The model under review builds one solid part; all positions refer to its coordinate system, in mm. A direction names the side the tool comes from. Give positions to 0.01 mm unless a question says otherwise; leave off trailing zeros. Order: outer loops, then holes, each group sorted by start corner. A loop starts at its lowest first (then second) coordinate and runs counter-clockwise, first axis right, second up.
```python
from build123d import *

# Parameters (mm, degrees)
ESQUISSE1_W                     = 10.5
ESQUISSE1_H                     = 1.75
ESQUISSE2_R                     = 4.45
BOSS_EXTRU_1_DEPTH              = 2.5
ESQUISSE3_R                     = 3.75
BOSS_EXTRU_2_DEPTH              = 0.5
DIAM_TRE_DU_PER_AGE_1_5_1_5_1_D = 1.5


with BuildPart() as part:
    # Esquisse1 → Révolution1 (revolve)
    with BuildSketch(Plane(origin=(0, 0, 0), x_dir=(-1, 0, 0), z_dir=(0, 0, -1)), mode=Mode.PRIVATE) as r_volution1_sk:
        with Locations((-5.25, -0.875)):
            Rectangle(ESQUISSE1_W, ESQUISSE1_H)
    revolve(r_volution1_sk.sketch.rotate(Axis((0, -1.75, 0), (0, 1, 0)), 270), axis=Axis((0, -1.75, 0), (0, 1, 0)))

    # Esquisse2 → Boss.-Extru.1 (add)
    with BuildSketch(Plane.XZ.offset(1.75)):
        with Locations(Location((0, 0, 0), (0, 0, 270))):
            Circle(ESQUISSE2_R)
    extrude(amount=BOSS_EXTRU_1_DEPTH)

    # Esquisse3 → Boss.-Extru.2 (add)
    with BuildSketch(Plane(origin=(0, 0, 0), x_dir=(-1, 0, 0), z_dir=(0, 1, 0))):
        with Locations(Location((0, 0, 0), (0, 0, 90))):
            Circle(ESQUISSE3_R)
    extrude(amount=BOSS_EXTRU_2_DEPTH)

    # Esquisse4 → Enlèvement de matière-Révolution1 (revolve, cut)
    with BuildSketch(Plane(origin=(0, 0, 0), x_dir=(-1, 0, 0), z_dir=(0, 0, -1)), mode=Mode.PRIVATE) as enl_vement_de_mati_re_r_volution1_sk:
        Polygon((-3, -4.5), (0, -4.5), (0, 0.5), (-3, 0.5), (-3, -0.5), (-1.500593113, -0.5), (-1.500593113, -1.5), (-3, -1.5), align=None)
    revolve(enl_vement_de_mati_re_r_volution1_sk.sketch.rotate(Axis((0, -4.5, 0), (0, 1, 0)), 270), axis=Axis((0, -4.5, 0), (0, 1, 0)), mode=Mode.SUBTRACT)

    # Diamètre du perçage Ø1.5 (1.5)1 (through all)
    with Locations(Plane(origin=(0, -1.75, 0), x_dir=(-1, 0, 0), z_dir=(0, -1, 0))):
        with Locations((-7, 0), (0, 7), (7, 0), (0, -7)):
            Hole(DIAM_TRE_DU_PER_AGE_1_5_1_5_1_D / 2)


solid = part.part
```
Item 1: Draft analysis for pull direction Z (two halves, no side actions). For faces 1 (the cylindrical face through (0.9, -0.01, 2.86)), 2 (the flat face through (3, 0.5, 1)), 3 (the cylindrical face through (3.01, -2.98, 3.28)), 4 (the flat face through (-1.3, -1.5, -1.3)), state which applies: released by +Z, released by -Z, zero draft, split by the parting line, or undercut.
Values found:
face 1: undercut
face 2: zero draft
face 3: split by the parting line
face 4: undercut
Item 2: Take a section at A-A (z = 0). Give the number of separate pieces and of enclosed holes in the cut face, and give its area (3 significant figures).
Values found:
separate pieces: 4
enclosed holes: 0
area: 32.0 mm2
Item 3: For line 1 (Z direction, x = 0.5, y = -1.4); line 2 (Y direction, x = 2.5, z = 8.5); line 3 (X direction, y = -2, z = 0), list the stretches that pass through material, from the lowest coordinate up.
Values found:
line 1: z = -10.49 to -7.56, -6.44 to -1.41, 1.41 to 6.44, 7.56 to 10.49
line 2: y = -1.75 to 0
line 3: x = -4.45 to -3, 3 to 4.45
Item 4: Clearance check with flat-ended pins moving along their axes: pin 1 Ø1.5 at (x, y) = (3.5, -1.5) entering from +Z; pin 2 Ø6 at (x, z) = (-7.5, 2.5) entering from -Y; pin 3 Ø5 at (x, z) = (0, 0) entering from +Y. State where each tip first meets the part, or that it passes through.
Values found:
pin 1: stops at z = 10.13
pin 2: stops at y = -1.75
pin 3: stops at y = -0.5
Item 5: Take a section at B-B (x = 6.5). Give the boundary of the cut face in (y, z), and give its area (3 significant figures).
Values found:
outline: (-1.75, -8.25) - (0, -8.25) - (0, -0.56) - (-1.75, -0.56) - close; (-1.75, 0.56) - (0, 0.56) - (0, 8.25) - (-1.75, 8.25) - close
area: 26.9 mm2
Item 6: Take a section at C-C (y = -1.1). Give the boundary of the cut face in (x, z), and give its area (3 significant figures).
Values found:
outline: circle Ø21 at (0, 0); hole circle Ø1.5 at (-7, 0); hole circle Ø3 at (0, 0); hole circle Ø1.5 at (0, -7); hole circle Ø1.5 at (0, 7); hole circle Ø1.5 at (7, 0)
area: 332 mm2
Item 7: For faces 5 (the flat face through (0, 0, 5)), 6 (the flat face through (0, -1.75, 5)), 7 (the cylindrical face through (3.2, -0.9, 10)), list the 3-axis set-ups (+Z, -Z, +X, -X, +Y, -Y) from which the entire face can be reached by the end or side of a thin tool; tool diameter is ignored.
Values found:
face 5: +Y
face 6: -Y
face 7: +Y, -Y
Item 8: Take a section at D-D (y = -3.55). Give the boundary of the cut face in (x, z), and give its area (3 significant figures).
Values found:
outline: circle Ø8.9 at (0, 0); hole circle Ø6 at (0, 0)
area: 33.9 mm2
